```python
from build123d import *

# Parameters (mm, degrees)
F1_DEPTH = 3.3528
F3_DEPTH = 3.3528
F4_D     = 3.6576


with BuildPart() as f1:
    # F0 (on Front) → F1 (new body)
    with BuildSketch(Plane.XZ):
        with BuildLine():
            Line((-256.0487464639, -118.0957335805), (-256.0487464639, -152.5127335805))
            Line((-256.0487464639, -152.5127335805), (226.5512535361, -152.5127335805))
            Line((226.5512535361, -152.5127335805), (226.5512535361, -118.0957335805))
            Line((226.5512535361, -118.0957335805), (216.2642535361, -118.0957335805))
            ThreePointArc((216.2642535361, -118.0957335805), (213.0892535361, -114.9207335805), (216.2642535361, -111.7457335805))
            Line((216.2642535361, -111.7457335805), (226.5512535361, -111.7457335805))
            Line((226.5512535361, -111.7457335805), (226.5512535361, -15.4797335805))
            Line((226.5512535361, -15.4797335805), (216.2642535361, -15.4797335805))
            ThreePointArc((216.2642535361, -15.4797335805), (213.0892535361, -12.3047335805), (216.2642535361, -9.1297335805))
            Line((216.2642535361, -9.1297335805), (226.5512535361, -9.1297335805))
            Line((226.5512535361, -9.1297335805), (226.5512535361, 25.2872664195))
            Line((226.5512535361, 25.2872664195), (-256.0487464639, 25.2872664195))
            Line((-256.0487464639, 25.2872664195), (-256.0487464639, -9.1297335805))
            Line((-256.0487464639, -9.1297335805), (-245.7617464639, -9.1297335805))
            ThreePointArc((-245.7617464639, -9.1297335805), (-242.5867464639, -12.3047335805), (-245.7617464639, -15.4797335805))
            Line((-245.7617464639, -15.4797335805), (-256.0487464639, -15.4797335805))
            Line((-256.0487464639, -15.4797335805), (-256.0487464639, -111.7457335805))
            Line((-256.0487464639, -111.7457335805), (-245.7617464639, -111.7457335805))
            ThreePointArc((-245.7617464639, -111.7457335805), (-242.5867464639, -114.9207335805), (-245.7617464639, -118.0957335805))
            Line((-245.7617464639, -118.0957335805), (-256.0487464639, -118.0957335805))
        make_face()
    extrude(amount=F1_DEPTH)

    # F2 (on face) → F3 (cut, through all)
    with BuildSketch(Plane.XZ.offset(3.3528)):
        with BuildLine():
            ThreePointArc((64.2454358226, 11.190272807), (62.3855638831, 15.6804008674), (57.8954358226, 17.5402728069))
            Line((57.8954358226, 17.5402728069), (-87.3925641774, 17.5402728068))
            ThreePointArc((-87.3925641774, 17.5402728068), (-91.8826922379, 15.6804008674), (-93.7425641774, 11.1902728068))
            Line((-93.7425641774, 11.1902728068), (-93.7425641774, -124.1917271931))
            ThreePointArc((-93.7425641774, -124.1917271931), (-91.882692238, -128.6818552537), (-87.3925641774, -130.5417271931))
            Line((-87.3925641774, -130.5417271931), (57.8954358225, -130.5417271931))
            ThreePointArc((57.8954358225, -130.5417271931), (62.3855638831, -128.6818552536), (64.2454358226, -124.1917271931))
            Line((64.2454358226, -124.1917271931), (64.2454358226, 11.190272807))
        make_face()
    extrude(amount=-F3_DEPTH, mode=Mode.SUBTRACT)

    # F4 (through all)
    with Locations(Plane.XZ.offset(3.3528)):
        with Locations((-98.0605641774, -126.2237271929), (68.5634358226, -126.2237271929), (68.5634358226, 12.2062728071), (-98.0605641774, 12.2062728071)):
            Hole(F4_D / 2)


solid = f1.part
```
The listing builds one solid part. Answer for the finished solid, in the listing's coordinates (mm). Coordinates: 2 decimals unless noted, no trailing zeros. Loops run counter-clockwise (first coordinate to the right, second up) from the corner with the lowest first, then second, coordinate; pieces in that order, holes last. Notation, with made-up numbers: (25.5, 50) - (46.5, 50) arc R21 cw to (46.5, 74) - close; hole circle Ø5 at (75.25, 86). An arc over 180 degrees is marked (long way). Write item = value, one per line.
1) Find the intervals of material crossed by line 1 along X through (y, z) = (-2.6, -74); line 2 along Z through (x, y) = (45, -0.05); line 3 along X through (y, z) = (-3.05, 15.5), in increasing order.
Responses:
line_1 = -256.05 to -93.74, 64.25 to 226.55
line_2 = -152.51 to -130.54, 17.54 to 25.29
line_3 = -256.05 to -92.06, 62.56 to 226.55
2) Section C-C (y = -2.6) is taken. Count the separate pieces of the cut face and the enclosed holes in it, plus the area to 3 significant figures.
Responses:
separate_pieces = 1
enclosed_holes = 5
area = 62,100 mm^2
3) Section A-A (z = -99.5) is taken. Determine the outline of the cut face in (x, y).
Responses:
outline = (-256.05, -3.35) - (-93.74, -3.35) - (-93.74, 0) - (-256.05, 0) - close; (64.25, -3.35) - (226.55, -3.35) - (226.55, 0) - (64.25, 0) - close
4) Section B-B (x = -53) is taken. Determine the outline of the cut face in (y, z).
Responses:
outline = (-3.35, -152.51) - (0, -152.51) - (0, -130.54) - (-3.35, -130.54) - close; (-3.35, 17.54) - (0, 17.54) - (0, 25.29) - (-3.35, 25.29) - close
